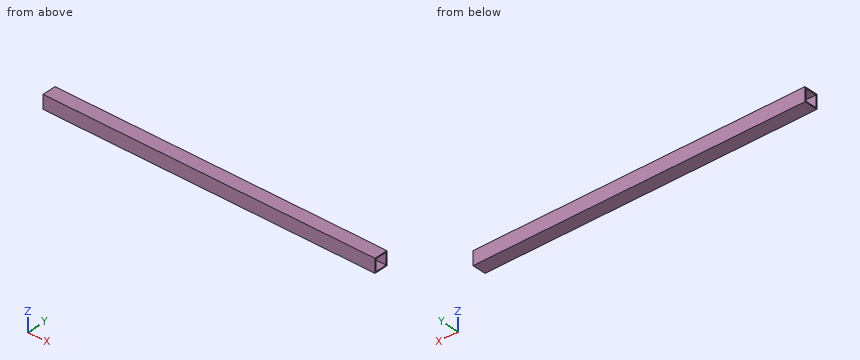
```python
from build123d import *

# Parameters (mm, degrees)
SKETCH024_W     = 1423.8
SKETCH024_H     = 38.1
PAD012_DEPTH    = 38.1
SKETCH025_W     = 32.7
SKETCH025_H     = 32.7
POCKET009_DEPTH = 1423.801
SKETCH030_W     = 499.970518
SKETCH030_H     = 38.1
POCKET011_DEPTH = 38.101


with BuildPart() as part:
    # Sketch024 (on Face1 of Binder005) → Pad012 (new body)
    with BuildSketch(Plane.XZ.offset(38.1)):
        with Locations((750, 1038.1)):
            Rectangle(SKETCH024_W, SKETCH024_H)
    extrude(amount=-PAD012_DEPTH)

    # Sketch025 (on Face1 of Pad012) → Pocket009 (cut, through all)
    with BuildSketch(Plane.YZ.offset(1461.9)):
        with Locations((-19.05, 1038.1)):
            Rectangle(SKETCH025_W, SKETCH025_H)
    extrude(amount=-POCKET009_DEPTH, mode=Mode.SUBTRACT)

    # Sketch030 (on Face3 of Pocket009) → Pocket011 (cut, through all)
    with BuildSketch(Plane.XZ.offset(38.1)):
        with Locations((288.085259, 1038.1)):
            Rectangle(SKETCH030_W, SKETCH030_H)
    extrude(amount=-POCKET011_DEPTH, mode=Mode.SUBTRACT)


with BuildPart() as part_1:
    # Body012 placement: moved
    add(part.part.moved(Location((0, 1538.1, 0))))


solid = part_1.part
```
Input: part model. Units: mm. Frame: model coordinates. Round coordinates to 2 decimals unless told otherwise and drop trailing zeros. Order: outer loops, then holes, each group sorted by start corner. A loop starts at its lowest first (then second) coordinate and runs counter-clockwise, first axis right, second up. Notation, with made-up numbers: (30.5, 40) - (88.5, 40) arc R34 ccw to (88.5, 74) - close; hole circle Ø1 at (-30.5, -6.5). An arc over 180 degrees is marked (long way). Answer in a Markdown table with one row per item.
Item 1: Section query C-C (x = 1011). Return the cut outline in (y, z), then the cut area to 3 significant figures.
Model answer:
| item | result |
|---|---|
| outline | (1500, 1019.05) - (1538.1, 1019.05) - (1538.1, 1057.15) - (1500, 1057.15) - close; hole (1502.7, 1021.75) - (1535.4, 1021.75) - (1535.4, 1054.45) - (1502.7, 1054.45) - close |
| area | 382 mm² |
Item 2: Section query B-B (z = 1037). Return the cut outline in (x, y).
Model answer:
| item | result |
|---|---|
| outline | (538.07, 1500) - (1461.9, 1500) - (1461.9, 1502.7) - (538.07, 1502.7) - close; (538.07, 1535.4) - (1461.9, 1535.4) - (1461.9, 1538.1) - (538.07, 1538.1) - close |
Item 3: Line query: line 1 (Y direction, x = 1157, z = 1045); line 2 (Z direction, x = 1179, y = 1508). Output: solid intervals per line, ascending.
Model answer:
| item | result |
|---|---|
| line 1 | y = 1500 to 1502.7, 1535.4 to 1538.1 |
| line 2 | z = 1019.05 to 1021.75, 1054.45 to 1057.15 |
Item 4: Section query A-A (y = 1513.5). Return the cut outline in (x, z), then the cut area to 3 significant figures.
Model answer:
| item | result |
|---|---|
| outline | (538.07, 1019.05) - (1461.9, 1019.05) - (1461.9, 1021.75) - (538.07, 1021.75) - close; (538.07, 1054.45) - (1461.9, 1054.45) - (1461.9, 1057.15) - (538.07, 1057.15) - close |
| area | 4,990 mm² |
